```python
from build123d import *

# Parameters (mm, degrees)
SKETCH1_W                         = 78
SKETCH1_H                         = 92.5
SKETCH1_R                         = 1.4
SKETCH1_W_2                       = 6
SKETCH1_H_2                       = 50
SKETCH1_W_3                       = 3
SKETCH1_H_3                       = 6
BASE_DEPTH                        = 5
SKETCH2_W                         = 71.5
SKETCH2_H                         = 84
PCB_CUTOUT_DEPTH                  = 2.5
F_1MM_EDGE_FILLETS_R              = 1
BASKET_CLAMP_MOUNTING_HOLES_REACH = 62.705
SKETCH3_R                         = 1.4


with BuildPart() as part:
    # Sketch1 → Base (new body)
    with BuildSketch(Plane(origin=(0, 0, 0), x_dir=(1, 0, 0), z_dir=(0, 1, 0))):
        Rectangle(SKETCH1_W, SKETCH1_H)
        with Locations(Location((-24.13, 12.05, 0), (0, 0, 270))):
            Circle(SKETCH1_R, mode=Mode.SUBTRACT)
        with Locations(Location((24.13, 13.32, 0), (0, 0, 270))):
            Circle(SKETCH1_R, mode=Mode.SUBTRACT)
        with Locations(Location((-8.89, -38.75, 0), (0, 0, 270))):
            Circle(SKETCH1_R, mode=Mode.SUBTRACT)
        with Locations((-30.5, -13.5)):
            Rectangle(SKETCH1_W_2, SKETCH1_H_2, mode=Mode.SUBTRACT)
        with Locations((30.5, -13.5)):
            Rectangle(SKETCH1_W_2, SKETCH1_H_2, mode=Mode.SUBTRACT)
        with Locations((31.75, 36.25)):
            Rectangle(SKETCH1_W_3, SKETCH1_H_3, mode=Mode.SUBTRACT)
        with Locations((-31.75, 36.25)):
            Rectangle(SKETCH1_W_3, SKETCH1_H_3, mode=Mode.SUBTRACT)
    extrude(amount=BASE_DEPTH)

    # Sketch2 → PCB Cutout (cut)
    with BuildSketch(Plane(origin=(0, 0, 0), x_dir=(1, 0, 0), z_dir=(0, 1, 0))):
        Rectangle(SKETCH2_W, SKETCH2_H)
    extrude(amount=PCB_CUTOUT_DEPTH, mode=Mode.SUBTRACT)

    # 1mm Edge Fillets
    f_1mm_edge_fillets_edges = [part.edges().sort_by_distance(p)[0] for p in [
        (39, 5, 0),
        (0, 5, -46.25),
        (-39, 5, 0),
        (-39, 2.5, -46.25),
        (39, 2.5, -46.25),
        (39, 2.5, 46.25),
        (-39, 2.5, 46.25),
        (0, 5, 46.25),
    ]]
    fillet(f_1mm_edge_fillets_edges, radius=F_1MM_EDGE_FILLETS_R)

    # Sketch3 → Basket Clamp Mounting Holes (cut, up to next)
    with BuildSketch(Plane(origin=(0, 5, 0), x_dir=(1, 0, 0), z_dir=(0, 1, 0)), mode=Mode.PRIVATE) as basket_clamp_mounting_holes_sk1:
        with Locations(Location((-4.5, -10, 0), (0, 0, 270))):
            Circle(SKETCH3_R)
    basket_clamp_mounting_holes_tool1 = extrude(basket_clamp_mounting_holes_sk1.sketch, amount=-BASKET_CLAMP_MOUNTING_HOLES_REACH, mode=Mode.PRIVATE) & part.part
    # Sketch3 → Basket Clamp Mounting Holes (cut, up to next)
    with BuildSketch(Plane(origin=(0, 5, 0), x_dir=(1, 0, 0), z_dir=(0, 1, 0)), mode=Mode.PRIVATE) as basket_clamp_mounting_holes_sk2:
        with Locations(Location((4.5, -10, 0), (0, 0, 270))):
            Circle(SKETCH3_R)
    basket_clamp_mounting_holes_tool2 = extrude(basket_clamp_mounting_holes_sk2.sketch, amount=-BASKET_CLAMP_MOUNTING_HOLES_REACH, mode=Mode.PRIVATE) & part.part
    add(basket_clamp_mounting_holes_tool1.solids().sort_by_distance((-4.5, 5, 10))[0], mode=Mode.SUBTRACT)
    add(basket_clamp_mounting_holes_tool2.solids().sort_by_distance((4.5, 5, 10))[0], mode=Mode.SUBTRACT)


solid = part.part
```
The listing builds one solid part. Answer for the finished solid, in the listing's coordinates (mm). A direction names the side the tool comes from. Round coordinates to 2 decimals unless told otherwise and drop trailing zeros. Loops run counter-clockwise (first coordinate to the right, second up) from the corner with the lowest first, then second, coordinate; pieces in that order, holes last. Notation, with made-up numbers: (39, -37.75) -> (62, -37.75) arc R15 cw to (62, -15.75) -> close; hole circle Ø4 at (18, -19). An arc over 180 degrees is marked (long way). Use one line per item in the form item = value.
1. The part is cut by section B-B on z = -2.5. Determine the outline of the cut face in (x, y), and give its area (3 significant figures).
Answer key:
outline = (-39, 0) -> (-35.75, 0) -> (-35.75, 2.5) -> (-33.5, 2.5) -> (-33.5, 5) -> (-38, 5) arc R1 ccw to (-39, 4) -> close; (-27.5, 2.5) -> (27.5, 2.5) -> (27.5, 5) -> (-27.5, 5) -> close; (33.5, 2.5) -> (35.75, 2.5) -> (35.75, 0) -> (39, 0) -> (39, 4) arc R1 ccw to (38, 5) -> (33.5, 5) -> close
area = 181 mm²
2. Find the intervals of material crossed by probe 1 along Z at (x, y) = (-29, 0.2); probe 2 along X at (y, z) = (3.35, 10); probe 3 along X at (y, z) = (3.5, 4.5), in increasing order. Write a range as [from, to].
Answer key:
probe_1 = [-46.25, -42], [42, 46.25]
probe_2 = [-39, -33.5], [-27.5, -5.9], [-3.1, 3.1], [5.9, 27.5], [33.5, 39]
probe_3 = [-39, -33.5], [-27.5, 27.5], [33.5, 39]
3. Flat-ended cylindrical pins translate along their axes: pin 1 Ø4.5 at (x, z) = (-24.13, -12.05) entering from -Y; pin 2 Ø3 at (x, y) = (30.5, 4.5) entering from +Z. Find the tip coordinate at first contact, or state that the pin passes through.
Answer key:
pin_1 = 2.5
pin_2 = 46.25
4. A tool of negligible diameter and unlimited length cuts with its end or side. For faces 3 (the flat face through (-33.5, 4, 14)), 4 (the flat face through (-38, 0, 0)), 5 (the flat face through (-1, 2.5, -1)), from which of +Z, -Z, +X, -X, +Y, -Y can it reach the whole face along a straight path? Write none if from no direction.
Answer key:
face_3 = +Y, -Y
face_4 = +Z, -Z, +X, -X, -Y
face_5 = -Y
5. The part is cut by section C-C on x = -12. Determine the outline of the cut face in (y, z), and give its area (3 significant figures).
Answer key:
outline = (0, -46.25) -> (4, -46.25) arc R1 ccw to (5, -45.25) -> (5, 45.25) arc R1 ccw to (4, 46.25) -> (0, 46.25) -> (0, 42) -> (2.5, 42) -> (2.5, -42) -> (0, -42) -> close
area = 252 mm²
6. For a pull along Z with two mould halves and no side action, classify faces 1 (the flat face through (30.25, 4, -36)), 2 (the flat face through (39, 2, 1)) as released by +Z, released by -Z, zero draft, split by the parting line, or undercut.
Answer key:
face_1 = undercut
face_2 = zero draft
7. The part is cut by section A-A on x = -24.13. Determine the outline of the cut face in (y, z), and give its area (3 significant figures).
Answer key:
outline = (0, -46.25) -> (4, -46.25) arc R1 ccw to (5, -45.25) -> (5, -13.45) -> (2.5, -13.45) -> (2.5, -42) -> (0, -42) -> close; (0, 42) -> (2.5, 42) -> (2.5, -10.65) -> (5, -10.65) -> (5, 45.25) arc R1 ccw to (4, 46.25) -> (0, 46.25) -> close
area = 245 mm²
